```python
from build123d import *

# Parameters (mm, degrees)
P_IDAT_VYSUNUT_M1_DEPTH  = 3
P_IDAT_VYSUNUT_M2_DEPTH  = 2
ZAOBLIT3_R               = 1
SKICA2_W                 = 4
SKICA2_H                 = 2
ODEBRAT_VYSUNUT_M1_DEPTH = 0.8
SKICA3_W                 = 4
SKICA3_H                 = 2
ODEBRAT_VYSUNUT_M2_DEPTH = 0.8


with BuildPart() as part:
    # Skica1 → P_idat vysunut_m1 (new body)
    with BuildSketch(Plane(origin=(0, 0, 0), x_dir=(1, 0, 0), z_dir=(0, 1, 0))):
        Polygon((-118.143750166, 15), (-118.143750166, 0), (-102.227105248, 19.278496169), (-95.473037065, 43.348863075), (-82.997228437, 47.003202833), (-48.112980408, 27.430537213), (-19, 0), (0, 0), (0, 15), (9.950504516, 11.37831254), (9.950504516, 24.27831254), (-10.5, 24.27831254), (-10.5, 37.37831254), (0, 33.55662508), (0, 69.224902673), (-39.317553332, 46.524902673), (-78.635106664, 69.224902673), (-118.143185584, 46.414902673), (-118.143185584, 33.5570142), (-107.643750166, 37.378496169), (-107.643750166, 24.278496169), (-128.093750166, 24.278496169), (-128.093750166, 11.378496169), align=None)
    extrude(amount=P_IDAT_VYSUNUT_M1_DEPTH)

    # Skica1_3 → P_idat vysunut_m2 (add)
    with BuildSketch(Plane(origin=(0, 0, 0), x_dir=(1, 0, 0), z_dir=(0, 1, 0))):
        Polygon((-102.227105248, 19.278496169), (-118.143750166, 0), (-19, 0), (-48.112980408, 27.430537213), (-82.997228437, 47.003202833), (-95.473037065, 43.348863075), align=None)
    extrude(amount=P_IDAT_VYSUNUT_M2_DEPTH)

    # Zaoblit3
    zaoblit3_edges = [part.edges().sort_by_distance(p)[0] for p in [
        (-10.5, 1.5, -24.27831254),
        (9.950504516, 1.5, -24.27831254),
        (9.950504516, 1.5, -11.37831254),
        (0, 1.5, -15),
        (-118.143750166, 1.5, -15),
        (-128.093750166, 1.5, -11.378496169),
        (-128.093750166, 1.5, -24.278496169),
        (-107.643750166, 1.5, -24.278496169),
        (-107.643750166, 1.5, -37.378496169),
        (-118.143185584, 1.5, -33.5570142),
        (0, 1.5, -33.55662508),
        (-10.5, 1.5, -37.37831254),
    ]]
    fillet(zaoblit3_edges, radius=ZAOBLIT3_R)

    # Skica2 → Odebrat vysunut_m1 (cut)
    with BuildSketch(Plane(origin=(0, 3, 0), x_dir=(1, 0, 0), z_dir=(0, 1, 0))):
        with Locations((-105.643750166, 28.314422166)):
            Rectangle(SKICA2_W, SKICA2_H)
    extrude(amount=-ODEBRAT_VYSUNUT_M1_DEPTH, mode=Mode.SUBTRACT)

    # Skica3 → Odebrat vysunut_m2 (cut)
    with BuildSketch(Plane(origin=(0, 3, 0), x_dir=(1, 0, 0), z_dir=(0, 1, 0))):
        with Locations((-12.5, 32.914238537)):
            Rectangle(SKICA3_W, SKICA3_H)
        with Locations((-12.5, 28.314238537)):
            Rectangle(SKICA3_W, SKICA3_H)
    extrude(amount=-ODEBRAT_VYSUNUT_M2_DEPTH, mode=Mode.SUBTRACT)


solid = part.part
```
Could you check a few things on this model? Use its own coordinates, in mm. A direction names the side the tool comes from. Round coordinates to 2 decimals unless told otherwise and drop trailing zeros. Loops run counter-clockwise (first coordinate to the right, second up) from the corner with the lowest first, then second, coordinate; pieces in that order, holes last.
Q1. Thinking about a two-plate mould opening in X: for faces 5 (the flat face through (-5.305, 1.479, -35.487)), 6 (the flat face through (-118.143, 1, -41)), 7 (the flat face through (-65.799, 2.493, -37.354)), 8 (the flat face through (9.951, 1, -18)), which applies, pulls with the +X half, pulls with the -X half, needs draft (parallel to the pull), parting line crosses it, or undercut?
Q2. Please list where these lines run through material, in increasing order: L1, parallel to Y at x = -65, z = -22; L2, parallel to Z at x = -111, y = 2.4; L3, parallel to X at y = 2.75, z = -32.5.
Q3. I want a section at C-C (z = -17.5). Write out the boundary of the cut face in (x, y), and give its area (3 significant figures).
Q4. I want a section at A-A (z = -59.5). Write out the boundary of the cut face in (x, y).
Q5. For P1, Ø0.9, axis at y = 1, z = -31.5, coming from the -X side; P2, Ø1, axis at x = -106, z = -28.5, coming from the +Y side; P3, Ø0.9, axis at y = 1.5, z = -5.5, coming from the +X side, each with a flat end and sliding along its axis, tell me the tip position at first contact or that it passes through.
Q6. On a 3-axis mill with a long thin cutter (end or side, diameter ignored), from which of +Z, -Z, +X, -X, +Y, -Y can I reach the whole of each face in a straight line? I mean faces 1 (the flat face through (4.92, 1.48, -13.21)), 2 (the flat face through (-107.644, 1, -31)), 3 (the flat face through (-98.897, 2.493, -31.145)), 4 (the flat face through (0, 1, -52)). Say none if no direction works.
Q7. I want a section at D-D (x = -68.5). Write out the boundary of the cut face in (y, z).
Answer below:
1. face 5: undercut
1. face 6: pulls with the -X half
1. face 7: undercut
1. face 8: pulls with the +X half
2. L1: y = 0 to 2
2. L2: z = -50.54 to -36.16, -24.28 to -8.65
2. L3: x = -107.64 to -98.52, -57.15 to -14.5
3. outline: (-128.09, 0) - (9.95, 0) - (9.95, 3) - (-37.57, 3) - (-37.57, 2) - (-103.7, 2) - (-103.7, 3) - (-128.09, 3) - close
3. area: 348 mm2
4. outline: (-95.48, 0) - (-61.79, 0) - (-61.79, 3) - (-95.48, 3) - close; (-16.84, 0) - (0, 0) - (0, 3) - (-16.84, 3) - close
5. P1: stops at x = -107.64
5. P2: stops at y = 2.2
5. P3: stops at x = 0
6. face 1: +Z, +Y, -Y
6. face 2: +Y, -Y
6. face 3: +Z, +Y
6. face 4: -Z, +X, +Y, -Y
7. outline: (0, -63.37) - (3, -63.37) - (3, -38.87) - (2, -38.87) - (2, 0) - (0, 0) - close
